For this review, take the finished solid that the model builds, in its own axes (mm). A direction names the side the tool comes from. Give positions to 0.01 mm unless a question says otherwise; leave off trailing zeros. Order: outer loops, then holes, each group sorted by start corner. A loop starts at its lowest first (then second) coordinate and runs counter-clockwise, first axis right, second up.
from build123d import *
from OCP.BRepFilletAPI import BRepFilletAPI_MakeChamfer

# Parameters (mm, degrees)
BOSS_EXTRUDE1_DEPTH = 34
SKETCH2_W           = 87
SKETCH2_H           = 38.5
BOSS_EXTRUDE2_DEPTH = 162
SKETCH3_W           = 65.25
SKETCH3_H           = 1.65
BOSS_EXTRUDE3_DEPTH = 8.86
FILLET1_R           = 1
CHAMFER1_SIZE2      = 1.5
CHAMFER1_SIZE       = 4.121216129
FILLET2_R           = 1.5
SKETCH4_W           = 24
SKETCH4_H           = 31
BOSS_EXTRUDE4_DEPTH = 3.75
CUT_EXTRUDE1_DEPTH  = 16.75
SKETCH6_W           = 4
SKETCH6_H           = 2
BOSS_EXTRUDE5_DEPTH = 11.75
SKETCH7_W           = 4
SKETCH7_H           = 2
BOSS_EXTRUDE6_DEPTH = 15.75
CHAMFER2_SIZE       = 0.7
CHAMFER2_SIZE2      = 1.923234194
FILLET3_R           = 0.5


with BuildPart() as part:
    # Sketch1 → Boss-Extrude1 (new body)
    with BuildSketch(Plane.XY):
        Polygon((42.75, 40), (82.75, 40), (82.75, 38.5), (87, 38.5), (87, 0), (0, 0), (0, 38.5), (42.75, 38.5), align=None)
    extrude(amount=-BOSS_EXTRUDE1_DEPTH)

    # Sketch2 → Boss-Extrude2 (add)
    with BuildSketch(Plane(origin=(0, 0, -34), x_dir=(-1, 0, 0), z_dir=(0, 0, -1))):
        with Locations((-43.5, 19.25)):
            Rectangle(SKETCH2_W, SKETCH2_H)
    extrude(amount=BOSS_EXTRUDE2_DEPTH)

    # Sketch3 → Boss-Extrude3 (add)
    with BuildSketch(Plane(origin=(0, 0, -196), x_dir=(-1, 0, 0), z_dir=(0, 0, -1))):
        with Locations((-42.375, 5.175)):
            Rectangle(SKETCH3_W, SKETCH3_H)
    extrude(amount=BOSS_EXTRUDE3_DEPTH)

    # Fillet1
    fillet1_edges = [part.edges().sort_by_distance(p)[0] for p in [
        (87, 19.25, 0),
        (0, 19.25, 0),
        (0, 19.25, -196),
        (87, 19.25, -196),
    ]]
    fillet(fillet1_edges, radius=FILLET1_R)

    # Chamfer1
    chamfer1_edges = [part.edges().sort_by_distance(p)[0] for p in [
        (62.75, 40, -34),
    ]]
    chamfer1_side = [part.faces().sort_by_distance(p)[0] for p in [
        (62.75, 40, -33.97),
    ]]
    chamfer(chamfer1_edges, length=CHAMFER1_SIZE - 0.0001, length2=CHAMFER1_SIZE2 - 0.0001, reference=chamfer1_side[0])  # a hair under: the kernel refuses the full size

    # Fillet2
    fillet2_edges = [part.edges().sort_by_distance(p)[0] for p in [
        (42.75, 40, -14.939441935),
        (82.75, 40, -14.939441935),
    ]]
    fillet(fillet2_edges, radius=FILLET2_R - 0.0001)  # a hair under: the kernel refuses the full size

    # Sketch4 → Boss-Extrude4 (add)
    with BuildSketch(Plane.XY):
        with Locations((18.5, 19.25)):
            Rectangle(SKETCH4_W, SKETCH4_H)
    extrude(amount=BOSS_EXTRUDE4_DEPTH)

    # Sketch5 → Cut-Extrude1 (cut)
    with BuildSketch(Plane.XY.offset(3.75)):
        with BuildLine():
            Line((27.2, 13.792640687), (27.2, 24.707359313))
            ThreePointArc((27.2, 24.707359313), (26.971638598, 25.85540961), (26.321320344, 26.828679656))
            Line((26.321320344, 26.828679656), (22.578679656, 30.571320344))
            ThreePointArc((22.578679656, 30.571320344), (21.60540961, 31.221638598), (20.457359313, 31.45))
            Line((20.457359313, 31.45), (12.8, 31.45))
            ThreePointArc((12.8, 31.45), (10.678679656, 30.571320344), (9.8, 28.45))
            Line((9.8, 28.45), (9.8, 10.05))
            ThreePointArc((9.8, 10.05), (10.678679656, 7.928679656), (12.8, 7.05))
            Line((12.8, 7.05), (20.457359313, 7.05))
            ThreePointArc((20.457359313, 7.05), (21.60540961, 7.278361402), (22.578679656, 7.928679656))
            Line((22.578679656, 7.928679656), (26.321320344, 11.671320344))
            ThreePointArc((26.321320344, 11.671320344), (26.971638598, 12.64459039), (27.2, 13.792640687))
        make_face()
    extrude(amount=-CUT_EXTRUDE1_DEPTH, mode=Mode.SUBTRACT)

    # Sketch6 → Boss-Extrude5 (add)
    with BuildSketch(Plane.XY.offset(-13)):
        with Locations((15.3, 25.95)):
            Rectangle(SKETCH6_W, SKETCH6_H)
        with Locations((15.3, 12.55)):
            Rectangle(SKETCH6_W, SKETCH6_H)
    extrude(amount=BOSS_EXTRUDE5_DEPTH)

    # Sketch7 → Boss-Extrude6 (add)
    with BuildSketch(Plane.XY.offset(-13)):
        with Locations((21.2, 19.25)):
            Rectangle(SKETCH7_W, SKETCH7_H)
    extrude(amount=BOSS_EXTRUDE6_DEPTH)

    # Chamfer2: one chamfer whose edges measure the first distance from different faces: ONE call of the kernel's chamfer builder (chamfer() names one face for all edges)
    chamfer2_edges_1 = [part.edges().sort_by_distance(p)[0] for p in [
        (17.3, 25.95, -1.25),
        (15.3, 26.95, -1.25),
        (13.3, 25.95, -1.25),
        (15.3, 24.95, -1.25),
    ]]
    chamfer2_side_1 = [part.faces().sort_by_distance(p)[0] for p in [
        (15.3, 25.95, -1.25),
    ]]
    chamfer2_edges_2 = [part.edges().sort_by_distance(p)[0] for p in [
        (17.3, 12.55, -1.25),
        (15.3, 13.55, -1.25),
        (13.3, 12.55, -1.25),
        (15.3, 11.55, -1.25),
    ]]
    chamfer2_side_2 = [part.faces().sort_by_distance(p)[0] for p in [
        (15.3, 12.55, -1.25),
    ]]
    chamfer2_edges_3 = [part.edges().sort_by_distance(p)[0] for p in [
        (21.2, 18.25, 2.75),
        (23.2, 19.25, 2.75),
        (21.2, 20.25, 2.75),
        (19.2, 19.25, 2.75),
    ]]
    chamfer2_side_3 = [part.faces().sort_by_distance(p)[0] for p in [
        (21.2, 19.25, 2.75),
    ]]
    chamfer2 = BRepFilletAPI_MakeChamfer(part.part.solid().wrapped)
    for e in chamfer2_edges_1:
        chamfer2.Add(CHAMFER2_SIZE, CHAMFER2_SIZE2, e.wrapped, chamfer2_side_1[0].wrapped)  # the first distance lies on this face
    for e in chamfer2_edges_2:
        chamfer2.Add(CHAMFER2_SIZE, CHAMFER2_SIZE2, e.wrapped, chamfer2_side_2[0].wrapped)  # the first distance lies on this face
    for e in chamfer2_edges_3:
        chamfer2.Add(CHAMFER2_SIZE, CHAMFER2_SIZE2, e.wrapped, chamfer2_side_3[0].wrapped)  # the first distance lies on this face
    add(Compound.cast(chamfer2.Shape()), mode=Mode.REPLACE)

    # Fillet3
    fillet3_edges = [part.edges().sort_by_distance(p)[0] for p in [
        (30.5, 3.75, 1.875),
        (30.5, 34.75, 1.875),
        (6.5, 34.75, 1.875),
        (6.5, 3.75, 1.875),
        (30.5, 19.25, 3.75),
        (18.5, 34.75, 3.75),
        (6.5, 19.25, 3.75),
        (18.5, 3.75, 3.75),
        (10.678679656, 7.928679656, 3.75),
        (16.628679656, 7.05, 3.75),
        (21.60540961, 7.278361402, 3.75),
        (24.45, 9.8, 3.75),
        (26.971638598, 12.64459039, 3.75),
        (27.2, 19.25, 3.75),
        (26.971638598, 25.85540961, 3.75),
        (24.45, 28.7, 3.75),
        (21.60540961, 31.221638598, 3.75),
        (16.628679656, 31.45, 3.75),
        (10.678679656, 30.571320344, 3.75),
        (9.8, 19.25, 3.75),
    ]]
    fillet(fillet3_edges, radius=FILLET3_R)


solid = part.part
1) We need section A-A on x = 37.5. Give the boundary of the cut face in (y, z).
Answer sheet:
outline: (0, -196) - (4.35, -196) - (4.35, -204.86) - (6, -204.86) - (6, -196) - (38.5, -196) - (38.5, 0) - (0, 0) - close
2) We need section C-C on z = -49. Give the boundary of the cut face in (x, y).
Answer sheet:
outline: (0, 0) - (87, 0) - (87, 38.5) - (0, 38.5) - close
3) Tool access review of faces 4 (the face through (24.52, 28.83, 3.6)), 5 (the face through (43, 4.35, -200)), 6 (the face through (62, 40, -15)), 7 (the face through (43, 6, -200)): name each direction out of +Z, -Z, +X, -X, +Y, -Y from which nothing blocks a thin tool from reaching the whole face with its end or side.
Answer sheet:
face 4: +Z
face 5: -Z, +X, -X, -Y
face 6: +Z, -Z, +X, -X, +Y
face 7: -Z, +X, -X, +Y
4) Clearance check with flat-ended pins moving along their axes: pin 1 (4.5 mm diameter, centred on x = 31, z = -199.5, fed in from -Y); pin 2 (1.8 mm diameter, centred on y = 5, z = -199, fed in from -X); pin 3 (8 mm diameter, centred on x = 72, y = 11, fed in from +Z). State where each tip first meets the part, or that it passes through.
Answer sheet:
pin 1: stops at y = 4.35
pin 2: stops at x = 9.75
pin 3: stops at z = 0
5) To check wall thickness, follow line 1 (Y direction, x = 46, z = -71.5); line 2 (Z direction, x = 42, y = 3); line 3 (Z direction, x = 17, y = 11). State the ranges of each line that lie inside material, in increasing order.
Answer sheet:
line 1: y = 0 to 38.5
line 2: z = -196 to 0
line 3: z = -196 to -13
6) Draft analysis for pull direction X (two halves, no side actions). For faces 1 (the face through (29, 19, 3.75)), 2 (the face through (87, 19, -97)), 3 (the face through (21, 18.25, -6)), state which applies: +X half, -X half, draft (parallel to the pull), parting line (faces both ways), or undercut.
Answer sheet:
face 1: draft
face 2: +X half
face 3: undercut
